The model under review builds one solid part; all positions refer to its coordinate system, in mm. Round coordinates to 2 decimals unless told otherwise and drop trailing zeros. Write each loop counter-clockwise with the first axis right and the second up, starting at its lowest first coordinate (ties: lowest second). Pieces come first, ordered by that corner, then holes. Notation, with made-up numbers: M 25,79 L 77,79 A10 cw 77,92 Z; hole C 83.5,58.5 d9. An arc over 180 degrees is marked long. Write item = value, one per line. Start each with the question number.
Item 1: For pin 1 Ø1 at (x, y) = (3.5, 3) entering from -Z; pin 2 Ø4 at (x, z) = (-58, -21.5) entering from +Y, all flat-tipped, find the tip position at first contact; note any pin that passes through.
Item 2: The part is to be moulded in two halves that separate along Y. For faces 1 (the flat face through (89.45, 1, 8)), 2 (the cylindrical face through (89.03, 2.56, -29.76)), 3 (the flat face through (1, 0, 0)), say which applies: +Y half, -Y half, draft (parallel to the pull), parting line (faces both ways), or undercut.
Item 3: Take a section at A-A, the plane y = 3.25. Give the number of separate pieces and of enclosed holes in the cut face, plus the area to 3 significant figures.
Item 4: Take a section at C-C, the plane x = -60. Give the boundary of the cut face in (y, z), plus the area to 3 significant figures.
Item 5: Take a section at B-B, the plane z = -12. Give the boundary of the cut face in (x, y), plus the area to 3 significant figures.
Item 6: To check wall thickness, follow line 1 along X through (y, z) = (3.25, 29.75); line 2 along Y through (x, z) = (87.7, 29.9); line 3 along Y through (x, z) = (-87, 29). State the ranges of each line that lie inside material, in increasing order.
Autodesk Inventor part; units mm, degrees
ref_plane "YZ Plane" through (0, 0, 0) normal (1, 0, 0) x (0, 1, 0)
ref_plane "XZ Plane" through (0, 0, 0) normal (0, 1, 0) x (-1, 0, 0)
ref_plane "XY Plane" through (0, 0, 0) normal (0, 0, 1) x (1, 0, 0)
sketch "Sketch1" plane through (0, 0, 0) normal (0, 1, 0) x (-1, 0, 0)
  line L0 (89.45, 32.5) -> (-89.45, 32.5)
  line L1 (-89.45, 32.5) -> (-89.45, -32.5)
  line L2 (-89.45, -32.5) -> (89.45, -32.5)
  line L3 (89.45, -32.5) -> (89.45, 32.5)
  line L4 (89.45, 32.5) -> (-89.45, -32.5) construction
  line L5 (-89.45, 32.5) -> (89.45, -32.5) construction
  point P0 (0, 0)
  dimension "d0" = 178.9
  dimension "d1" = 65
extrude "Extrusion1" add sketch "Sketch1" along normal blind 1.5
sketch "Sketch2" plane through (0, 1.5, 0) normal (0, 1, 0) x (1, 0, 0)
  line L0 (89.45, -32.5) -> (89.45, 32.5)
  line L1 (-89.45, -29.75) -> (89.45, -29.75)
  line L2 (89.45, -29.75) -> (89.45, 29.75)
  line L3 (89.45, 29.75) -> (-89.45, 29.75)
  line L4 (-89.45, 29.75) -> (-89.45, -29.75)
  line L5 (-89.45, -29.75) -> (89.45, 29.75) construction
  line L6 (89.45, -29.75) -> (-89.45, 29.75) construction
  line L7 (89.45, 29.75) -> (85.95, 29.75)
  line L8 (85.95, 29.75) -> (85.95, 30.25)
  line L9 (85.95, 30.25) -> (89.45, 30.25)
  line L10 (89.45, 30.25) -> (89.45, 29.75)
  line L11 (85.95, 29.75) -> (85.95, 29.25)
  line L12 (85.95, 29.25) -> (89.45, 29.25)
  line L13 (89.45, 29.25) -> (89.45, 29.75)
  line L14 (0, 0) -> (0, 29.75)
  line L15 (0, 0) -> (37, 0)
  line L16 (-89.45, 29.75) -> (-85.95, 29.75)
  line L17 (-85.95, 29.75) -> (-85.95, 30.25)
  line L18 (-85.95, 30.25) -> (-89.45, 30.25)
  line L19 (-89.45, 30.25) -> (-89.45, 29.75)
  line L20 (-85.95, 29.75) -> (-85.95, 29.25)
  line L21 (-85.95, 29.25) -> (-89.45, 29.25)
  line L22 (-89.45, 29.25) -> (-89.45, 29.75)
  line L23 (89.45, -29.75) -> (85.95, -29.75)
  line L24 (85.95, -29.75) -> (85.95, -30.25)
  line L25 (85.95, -30.25) -> (89.45, -30.25)
  line L26 (89.45, -30.25) -> (89.45, -29.75)
  line L27 (85.95, -29.75) -> (85.95, -29.25)
  line L28 (85.95, -29.25) -> (89.45, -29.25)
  line L29 (89.45, -29.25) -> (89.45, -29.75)
  line L30 (-89.45, -29.75) -> (-85.95, -29.75)
  line L31 (-85.95, -29.75) -> (-85.95, -30.25)
  line L32 (-89.45, -30.25) -> (-89.45, -29.75)
  line L33 (-85.95, -29.75) -> (-85.95, -29.25)
  line L34 (-85.95, -29.25) -> (-89.45, -29.25)
  line L35 (-89.45, -29.25) -> (-89.45, -29.75)
  line L36 (-85.95, -30.25) -> (-89.45, -30.25)
  dimension "d4" = 59.5
  dimension "d5" = 3.5
  dimension "d6" = 0.5
extrude "Extrusion2" add sketch "Sketch2" along normal blind 3.5 contours L25 L24 L1 L0 | L1 L27 L28 L0 | L12 L11 L3 L0 | L31 L36 L32 L1 | L1 L4 L34 L33 | L3 L8 L9 L0 | L4 L3 L20 L21 | L3 L19 L18 L17
hole "Hole1" at (-87.7, 3.25, 30.25) direction (0, 0, -1) diameter 3 end through all
hole "Hole2" at (87.7, 3.25, 30.25) direction (0, 0, -1) diameter 3 end through all
properties part number "Bumper big"
Response values:
q1.pin_1 = through
q1.pin_2 = 1.5
q2.face_1 = draft
q2.face_2 = undercut
q2.face_3 = -Y half
q3.separate_pieces = 8
q3.enclosed_holes = 0
q3.area = 2.00 mm2
q4.outline = M 0,-32.5 L 1.5,-32.5 L 1.5,32.5 L 0,32.5 Z
q4.area = 97.5 mm2
q5.outline = M -89.45,0 L 89.45,0 L 89.45,1.5 L -89.45,1.5 Z
q5.area = 268 mm2
q6.line_1 = -89.45 to -89.2, -86.2 to -85.95, 85.95 to 86.2, 89.2 to 89.45
q6.line_2 = 0 to 1.75, 4.75 to 5
q6.line_3 = 0 to 1.5
